Model file for the job. Use its own axes, mm. Face numbers are marked on the shaded views. A direction names the side the tool comes from. Give positions to 0.01 mm unless a question says otherwise; leave off trailing zeros. Loops run counter-clockwise (first coordinate to the right, second up) from the corner with the lowest first, then second, coordinate; pieces in that order, holes last. Notation, with made-up numbers: M -9.5,80.25 L -0.5,80.25 A24 ccw -0.5,90.25 Z; hole C 72,73.25 d10. An arc over 180 degrees is marked long. Answer in a Markdown table with one row per item.
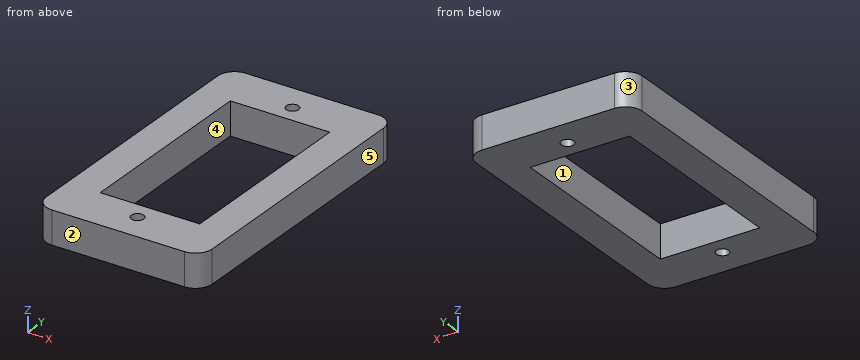
```python
from build123d import *

# Parameters (mm, degrees)
SKIZZE1_W                       = 20
SKIZZE1_H                       = 35
SKIZZE1_W_2                     = 12
SKIZZE1_H_2                     = 23.5
GRUNDPLATTE_DEPTH               = 4
SKIZZE2_R                       = 0.75
SCHNITT_LINEAR_AUSTRAGEN1_DEPTH = 21.548722588
VERRUNDUNG1_R                   = 2


with BuildPart() as part:
    # Skizze1 → Grundplatte (new body)
    with BuildSketch(Plane.XY):
        Rectangle(SKIZZE1_W, SKIZZE1_H)
        Rectangle(SKIZZE1_W_2, SKIZZE1_H_2, mode=Mode.SUBTRACT)
    extrude(amount=GRUNDPLATTE_DEPTH)

    # Skizze2 → Schnitt-Linear austragen1 (cut, through all)
    with BuildSketch(Plane.XY.offset(4)):
        with Locations((0, 14)):
            Circle(SKIZZE2_R)
        with Locations(Location((0, -14, 0), (0, 0, 180))):
            Circle(SKIZZE2_R)
    extrude(amount=-SCHNITT_LINEAR_AUSTRAGEN1_DEPTH, mode=Mode.SUBTRACT)

    # Verrundung1
    verrundung1_edges = [part.edges().sort_by_distance(p)[0] for p in [
        (10, -17.5, 2),
        (-10, -17.5, 2),
        (-10, 17.5, 2),
        (10, 17.5, 2),
    ]]
    fillet(verrundung1_edges, radius=VERRUNDUNG1_R)


solid = part.part
```
Q1. Saw through at D-D (x = -5.5). Give the cut face in (y, z), and give its area (3 significant figures).
Reported:
| item | result |
|---|---|
| outline | M -17.5,0 L -11.75,0 L -11.75,4 L -17.5,4 Z; M 11.75,0 L 17.5,0 L 17.5,4 L 11.75,4 Z |
| area | 46.0 mm² |
Q2. Saw through at B-B (x = 0). Give the cut face in (y, z).
Reported:
| item | result |
|---|---|
| outline | M -17.5,0 L -14.75,0 L -14.75,4 L -17.5,4 Z; M -13.25,0 L -11.75,0 L -11.75,4 L -13.25,4 Z; M 11.75,0 L 13.25,0 L 13.25,4 L 11.75,4 Z; M 14.75,0 L 17.5,0 L 17.5,4 L 14.75,4 Z |
Q3. Saw through at C-C (z = 1.55). Give the cut face in (x, y).
Reported:
| item | result |
|---|---|
| outline | M -10,-15.5 A2 ccw -8,-17.5 L 8,-17.5 A2 ccw 10,-15.5 L 10,15.5 A2 ccw 8,17.5 L -8,17.5 A2 ccw -10,15.5 Z; hole M -6,-11.75 L 6,-11.75 L 6,11.75 L -6,11.75 Z; hole C 0,-14 d1.5; hole C 0,14 d1.5 |
Q4. Drop a flat-ended pin along its axis: pin 1 (0.9 mm diameter, centred on x = 0, y = -14, fed in from +Z). Give the stop position or say it passes through.
Reported:
| item | result |
|---|---|
| pin 1 | through |
Q5. Mould opens along Y. For the marked faces 1, 2 and 3 say: released by +Y, released by -Y, zero draft, split by the parting line, or undercut.
Reported:
| item | result |
|---|---|
| face 1 | undercut |
| face 2 | released by -Y |
| face 3 | released by +Y |
Q6. Probe probe 1 along Y at (x, z) = (0, 0.9); probe 2 along Y at (x, z) = (-5.25, 1.45); probe 3 along X at (y, z) = (-14, 2.9). List the from-to ranges inside material, lowest first.
Reported:
| item | result |
|---|---|
| probe 1 | -17.5 to -14.75, -13.25 to -11.75, 11.75 to 13.25, 14.75 to 17.5 |
| probe 2 | -17.5 to -11.75, 11.75 to 17.5 |
| probe 3 | -10 to -0.75, 0.75 to 10 |
Q7. Saw through at A-A (y = -14). Give the cut face in (x, z).
Reported:
| item | result |
|---|---|
| outline | M -10,0 L -0.75,0 L -0.75,4 L -10,4 Z; M 0.75,0 L 10,0 L 10,4 L 0.75,4 Z |
Q8. 3-axis set-ups, long thin cutter, end or side, ignore diameter. For the marked faces 4 and 5: which of +Z, -Z, +X, -X, +Y, -Y reach the whole face in a straight line?
Reported:
| item | result |
|---|---|
| face 4 | +Z, -Z |
| face 5 | +Z, -Z, +X, +Y, -Y |
